CAD build for the part. Positions are in the model's coordinates, mm. Face numbers are marked on the shaded views. A direction names the side the tool comes from. Coordinates: 2 decimals unless noted, no trailing zeros. Loops run counter-clockwise (first coordinate to the right, second up) from the corner with the lowest first, then second, coordinate; pieces in that order, holes last. Notation, with made-up numbers: (69.25, -34) -> (108.25, -34) arc R16 cw to (108.25, -10) -> close; hole circle Ø1 at (18, 31). An arc over 180 degrees is marked (long way). Write each question's results on one line, items separated by ' | '.
from build123d import *

# Parameters (mm, degrees)
SKETCH1_W               = 85
SKETCH1_H               = 25
BOSS_EXTRUDE1_DEPTH     = 3
SKETCH3_R               = 1.75
CUT_EXTRUDE2_DEPTH      = 45.401576549
FILLET2_R               = 2
SKETCH4_W               = 5
SKETCH4_H               = 20
BOSS_EXTRUDE2_DEPTH     = 25
FILLET3_R               = 10
CUT_EXTRUDE3_DEPTH      = 59.653644388
CUT_EXTRUDE3_DEPTH_BACK = 59.653644388
SKETCH5_R               = 2.75
CUT_EXTRUDE4_DEPTH      = 2.5
CHAMFER1_SIZE           = 2


with BuildPart() as part:
    # Sketch1 → Boss-Extrude1 (new body)
    with BuildSketch(Plane(origin=(0, 0, 0), x_dir=(1, 0, 0), z_dir=(0, 1, 0))):
        Rectangle(SKETCH1_W, SKETCH1_H)
    extrude(amount=BOSS_EXTRUDE1_DEPTH)

    # Sketch3 → Cut-Extrude2 (cut, through all)
    with BuildSketch(Plane(origin=(0, 3, 0), x_dir=(1, 0, 0), z_dir=(0, 1, 0))):
        with Locations(Location((-38.5, 8.5, 0), (0, 0, 270))):
            Circle(SKETCH3_R)
        with Locations(Location((38.5, 8.5, 0), (0, 0, 90))):
            Circle(SKETCH3_R)
        with Locations(Location((-29, -5, 0), (0, 0, 270))):
            Circle(SKETCH3_R)
        with Locations(Location((29, -5, 0), (0, 0, 90))):
            Circle(SKETCH3_R)
    extrude(amount=-CUT_EXTRUDE2_DEPTH, mode=Mode.SUBTRACT)

    # Fillet2
    fillet2_edges = [part.edges().sort_by_distance(p)[0] for p in [
        (-42.5, 1.5, -12.5),
        (42.5, 1.5, -12.5),
        (42.5, 1.5, 12.5),
        (-42.5, 1.5, 12.5),
    ]]
    fillet(fillet2_edges, radius=FILLET2_R)

    # Sketch4 → Boss-Extrude2 (add)
    with BuildSketch(Plane(origin=(0, 3, 0), x_dir=(1, 0, 0), z_dir=(0, 1, 0))):
        with Locations((-5, 0)):
            Rectangle(SKETCH4_W, SKETCH4_H)
        with Locations((5, 0)):
            Rectangle(SKETCH4_W, SKETCH4_H)
    extrude(amount=BOSS_EXTRUDE2_DEPTH)

    # Fillet3
    fillet3_edges = [part.edges().sort_by_distance(p)[0] for p in [
        (5, 28, 10),
        (5, 28, -10),
        (-5, 28, -10),
        (-5, 28, 10),
    ]]
    fillet(fillet3_edges, radius=FILLET3_R - 0.0001)  # a hair under: the kernel refuses the full size

    # Sketch5 → Cut-Extrude3 (cut, two sides: drawn at the far end of the back side and taken through both)
    with BuildSketch(Plane.ZY.offset(7.5).offset(-CUT_EXTRUDE3_DEPTH_BACK)):
        with Locations((0, 18)):
            Circle(SKETCH5_R)
    extrude(amount=CUT_EXTRUDE3_DEPTH + CUT_EXTRUDE3_DEPTH_BACK, mode=Mode.SUBTRACT)

    # Sketch6 → Cut-Extrude4 (cut)
    with BuildSketch(Plane(origin=(7.5, 0, 0), x_dir=(0, 0, -1), z_dir=(1, 0, 0))):
        Polygon((0, 13.236860279), (4.125, 15.61843014), (4.125, 20.38156986), (0, 22.763139721), (-4.125, 20.38156986), (-4.125, 15.61843014), align=None)
    extrude(amount=-CUT_EXTRUDE4_DEPTH, mode=Mode.SUBTRACT)

    # Chamfer1
    chamfer1_edges = [part.edges().sort_by_distance(p)[0] for p in [
        (-5, 3, -10),
        (-5, 3, 10),
        (5, 3, -10),
        (5, 3, 10),
    ]]
    chamfer(chamfer1_edges, length=CHAMFER1_SIZE)


solid = part.part
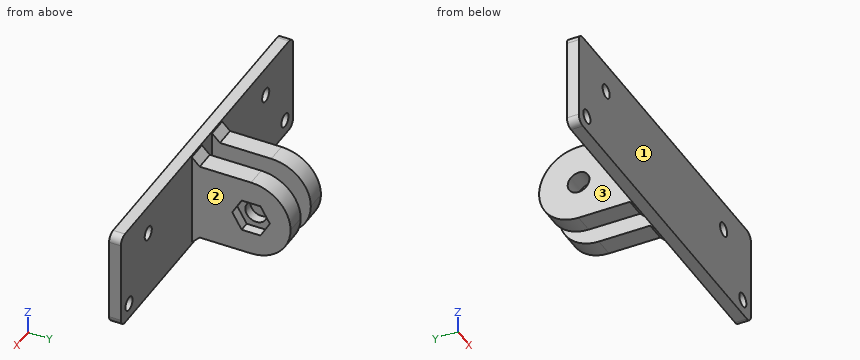
1) Slice it at C-C (z = -8.5). Write the cut outline in (x, y), then the cut area to 3 significant figures.
Outcome:
outline: (-42.5, 0) -> (-40.25, 0) -> (-40.25, 3) -> (-42.5, 3) -> close; (-36.75, 0) -> (36.75, 0) -> (36.75, 3) -> (7.5, 3) -> (7.5, 23.27) -> (2.5, 23.27) -> (2.5, 3) -> (-2.5, 3) -> (-2.5, 23.27) -> (-7.5, 23.27) -> (-7.5, 3) -> (-36.75, 3) -> close; (40.25, 0) -> (42.5, 0) -> (42.5, 3) -> (40.25, 3) -> close | area: 437 mm^2
2) Slice it at B-B (y = 9.25). Write the cut outline in (x, z), then the cut area to 3 significant figures.
Outcome:
outline: (-7.5, -10) -> (-2.5, -10) -> (-2.5, 10) -> (-7.5, 10) -> close; (2.5, -10) -> (7.5, -10) -> (7.5, 10) -> (2.5, 10) -> close | area: 200 mm^2
3) Pin check, flat tips, straight feed: pin 1 (4.5 mm diameter, centred on x = -38.5, z = -8.5, fed in from -Y); pin 2 (4 mm diameter, centred on x = 38.5, z = -8.5, fed in from +Y); pin 3 (7.5 mm diameter, centred on x = -2, z = 6, fed in from +Y); pin 4 (5.5 mm diameter, centred on x = 5.5, y = 14.5, fed in from +Z). Stop position of each tip, or through.
Outcome:
pin 1: stops at y = 0 | pin 2: stops at y = 3 | pin 3: stops at y = 27.74 | pin 4: stops at z = 10
4) Slice it at D-D (y = 16.5). Write the cut outline in (x, z) (3 decimals).
Outcome:
outline: (-7.5, -10) -> (-2.5, -10) -> (-2.5, -2.305) -> (-7.5, -2.305) -> close; (-7.5, 2.305) -> (-2.5, 2.305) -> (-2.5, 10) -> (-7.5, 10) -> close; (2.5, -10) -> (7.5, -10) -> (7.5, -4.125) -> (5, -4.125) -> (5, -2.305) -> (2.5, -2.305) -> close; (2.5, 2.305) -> (5, 2.305) -> (5, 4.125) -> (7.5, 4.125) -> (7.5, 10) -> (2.5, 10) -> close
5) Which spindle directions (+Z, -Z, +X, -X, +Y, -Y) get a long thin tool onto all of the face, cutting with end or side? Do the marked faces 1, 2 and 3. Say none if no direction does.
Outcome:
face 1: +Z, -Z, +X, -X, -Y | face 2: +Z, -Z, +X, +Y | face 3: +Z, -Z, -X, +Y
6) Drill centre lines: L1, parallel to X at y = 1.7, z = 5; L2, parallel to Z at x = 29, y = 1.8; L3, parallel to Y at x = -4.45, z = 0. Where is each one in solid material? Low to high. Write a range as from..to.
Outcome:
L1: x = -42.5..-30.75, -27.25..27.25, 30.75..42.5 | L2: z = -12.5..3.25, 6.75..12.5 | L3: y = 0..15.25, 20.75..28
7) Slice it at A-A (x = 29). Write the cut outline in (y, z).
Outcome:
outline: (0, -12.5) -> (3, -12.5) -> (3, 3.25) -> (0, 3.25) -> close; (0, 6.75) -> (3, 6.75) -> (3, 12.5) -> (0, 12.5) -> close
